Autodesk Inventor part; units mm, degrees
ref_plane "YZ Plane" through (0, 0, 0) normal (1, 0, 0) x (0, 1, 0)
ref_plane "XZ Plane" through (0, 0, 0) normal (0, 1, 0) x (-1, 0, 0)
ref_plane "XY Plane" through (0, 0, 0) normal (0, 0, 1) x (1, 0, 0)
sketch "Sketch1" plane through (0, 0, 0) normal (0, 0, 1) x (1, 0, 0)
  arc A0 (-1.778, 0) -> (1.778, 0) centre (0, 0) ccw
  line L0 (-1.778, 0) -> (-1.778, 3.81)
  line L1 (-1.778, 3.81) -> (1.778, 3.81)
  line L2 (1.778, 3.81) -> (1.778, 0)
  dimension "d0" = 3.556
  dimension "d1" = 3.81
extrude "Extrusion1" add sketch "Sketch1" along normal blind 0.5588
hole "Hole1" at (0, 0, 0.5588) direction (0, 0, -1) diameter 1.143 end through all
sketch "Sketch3" plane through (0, 0, 0) normal (1, 0, 0) x (0, 1, 0)
  line L0 (-0.5908, 1.8288) -> (-1.27, 1.8288)
  line L1 (-1.27, 1.8288) -> (-1.27, 1.7018)
  line L2 (0, 0.5588) -> (-1.778, 0.5588)
  line L3 (0, 1.8288) -> (0, 0.5588)
  line L4 (-0.5908, 0.5588) -> (-0.5908, 1.8288)
  line L5 (-1.27, 1.7018) -> (-0.7178, 1.7018)
  line L6 (0.5715, 0) -> (-0.5715, 0)
  line L7 (-0.5715, 0.5588) -> (0.5715, 0.5588)
  line L8 (-0.7178, 1.7018) -> (-0.7178, 0.5588)
  line L9 (-0.7178, 0.5588) -> (-0.5908, 0.5588)
  point P0 (0, 0)
  dimension "d21" = 0.127
  dimension "d22" = 1.27
revolve "Revolution1" add sketch "Sketch3" angle 360 about axis through (0, 0, 1.8288) along (0, 0, -1)
sketch "Sketch4" plane through (0, 0, 1.8288) normal (0, 0, 1) x (1, 0, 0)
  circle A0 centre (0, 0) radius 1.27
  line L0 (-0.127, 0.3054) -> (0.127, 0.3054)
  line L1 (0.127, 0.3054) -> (0.127, 1.3789)
  line L2 (0.127, 1.3789) -> (-0.127, 1.3789)
  line L3 (-0.127, 1.3789) -> (-0.127, 0.3054)
  line L4 (-0.328, 0.0427) -> (-0.201, 0.2627)
  line L5 (-0.201, 0.2627) -> (-1.1307, 0.7994)
  line L6 (-1.1307, 0.7994) -> (-1.2577, 0.5795)
  line L7 (-1.2577, 0.5795) -> (-0.328, 0.0427)
  line L8 (-0.201, -0.2627) -> (-0.328, -0.0427)
  line L9 (-0.328, -0.0427) -> (-1.2577, -0.5795)
  line L10 (-1.2577, -0.5795) -> (-1.1307, -0.7994)
  line L11 (-1.1307, -0.7994) -> (-0.201, -0.2627)
  line L12 (0.127, -0.3054) -> (-0.127, -0.3054)
  line L13 (-0.127, -0.3054) -> (-0.127, -1.3789)
  line L14 (-0.127, -1.3789) -> (0.127, -1.3789)
  line L15 (0.127, -1.3789) -> (0.127, -0.3054)
  line L16 (0.328, -0.0427) -> (0.201, -0.2627)
  line L17 (0.201, -0.2627) -> (1.1307, -0.7994)
  line L18 (1.1307, -0.7994) -> (1.2577, -0.5795)
  line L19 (1.2577, -0.5795) -> (0.328, -0.0427)
  line L20 (0.201, 0.2627) -> (0.328, 0.0427)
  line L21 (0.328, 0.0427) -> (1.2577, 0.5795)
  line L22 (1.2577, 0.5795) -> (1.1307, 0.7994)
  line L23 (1.1307, 0.7994) -> (0.201, 0.2627)
  dimension "d24" = 0.254
  dimension "d25" = 0.127
  dimension "d28" = 360
extrude "Extrusion2" cut sketch "Sketch4" against normal blind 0.0508 contours L21 L20 L23 A0 | A0 L23 L22 L21 | L19 L18 L17 A0 | A0 L17 L16 L19 | L1 L0 L3 A0 | A0 L3 L2 L1 | L15 L14 L13 A0 | A0 L13 L12 L15 | L5 L4 L7 A0 | A0 L7 L6 L5 | L11 L10 L9 A0 | A0 L9 L8 L11
sketch "Sketch5" plane through (0, 0, 0.5588) normal (0, 0, 1) x (1, 0, 0)
  arc A0 (-1.778, 0) -> (1.778, 0) centre (0, 0) ccw
  line L0 (1.778, 3.81) -> (-1.778, 3.81)
  line L1 (-0.4953, 3.81) -> (0.4953, 3.81)
  line L2 (0.4953, 3.81) -> (0.4953, 8.001)
  line L3 (0.4953, 8.001) -> (-0.4953, 8.001)
  line L4 (-0.4953, 8.001) -> (-0.4953, 3.81)
  dimension "d32" = 4.191
  dimension "d33" = 0.9906
  dimension "d34" = 0.4953
extrude "Extrusion3" add sketch "Sketch5" against normal up to surface (0.5588 mm away)
chamfer "Chamfer1" distance 0.0508 distance2 0.762 1 edges at (0.4953, 8.001, 0.2794) measured on face at (0.1651, 8.001, 0.3725)
chamfer "Chamfer2" distance 0.762 distance2 0.0508 1 edges at (-0.4953, 8.001, 0.2794) measured on face at (-0.4953, 6.604, 0.3725)
fillet "Fillet2" radius 0.127 2 edges at (0.4445, 8.001, 0.2794) (-0.4445, 8.001, 0.2794)
sketch "Sketch6" plane through (0, 0, 0) normal (0, 0, -1) x (-1, 0, 0)
  arc A0 (-1.778, 0) -> (1.778, 0) centre (0, 0) ccw
  point P0 (0, 2.54)
  dimension "d45" = 2.54
hole "Hole2" at (0, 2.54, 0) direction (0, 0, 1) diameter 1.143 end through all
equation "\"d25\" = 0.5 * d24"
equation "\"d34\" = 0.5 * d33"
properties part number "Potenciometro - Pata"
Work out the finished part from the listing and answer in its coordinate system (mm). Give positions to 0.01 mm unless a question says otherwise; leave off trailing zeros. Loops run counter-clockwise (first coordinate to the right, second up) from the corner with the lowest first, then second, coordinate; pieces in that order, holes last. Notation, with made-up numbers: (-6.75, 44.25) -> (13.25, 44.25) arc R9 ccw to (13.25, 56.25) -> close; hole circle Ø7 at (81.25, 16.25). An arc over 180 degrees is marked (long way). Use a Markdown table: item, result. Add a question column.
1) The part is cut by section B-B, the plane x = 0. Count the separate pieces of the cut face and the enclosed holes in it, plus the area to 3 significant figures.
2) The part is cut by section C-C, the plane z = 0.25. Determine the outline of the cut face in (x, y).
3) Consider line 1 along Y through (x, z) = (0, 0.15); line 2 along X through (y, z) = (2.54, 0.35); line 3 along Z through (x, y) = (-0.6, 1.5). Determine where each line is inside the solid, lowest interval first.
4) The part is cut by section D-D, the plane z = 1.6. Determine the outline of the cut face in (x, y), plus the area to 3 significant figures.
5) Each of these flat-tipped pins is pushed along its axis until it touches: P1, Ø1, axis at x = -1.5, z = 0, coming from the +Y side; P2, Ø1.5, axis at x = 0, y = 7, coming from the +Z side. Where does it stop, or does it pass through?
6) The part is cut by section A-A, the plane y = 2.54. Determine the outline of the cut face in (x, z).
Reported:
| question | item | result |
|---|---|---|
| 1 | separate pieces | 3 |
| 1 | enclosed holes | 0 |
| 1 | area | 4.58 mm^2 |
| 2 | outline | (-1.78, 0) arc R1.78 ccw to (1.78, 0) -> (1.78, 3.81) -> (0.5, 3.81) -> (0.5, 7.24) -> (0.45, 7.88) arc R0.13 ccw to (0.33, 8) -> (-0.33, 8) arc R0.13 ccw to (-0.45, 7.88) -> (-0.5, 7.24) -> (-0.5, 3.81) -> (-1.78, 3.81) -> close; hole circle Ø1.14 at (0, 0); hole circle Ø1.14 at (0, 2.54) |
| 3 | line 1 | y = -1.78 to -0.57, 0.57 to 1.97, 3.11 to 8 |
| 3 | line 2 | x = -1.78 to -0.57, 0.57 to 1.78 |
| 3 | line 3 | z = 0 to 0.56 |
| 4 | outline | circle Ø1.44 at (0, 0); hole circle Ø1.18 at (0, 0) |
| 4 | area | 0.522 mm^2 |
| 5 | P1 | stops at y = 3.81 |
| 5 | P2 | stops at z = 0.56 |
| 6 | outline | (-1.78, 0) -> (-0.57, 0) -> (-0.57, 0.56) -> (-1.78, 0.56) -> close; (0.57, 0) -> (1.78, 0) -> (1.78, 0.56) -> (0.57, 0.56) -> close |
